Work out the finished part from the listing and answer in its coordinate system (mm). A direction names the side the tool comes from. Coordinates: 2 decimals unless noted, no trailing zeros. Loops run counter-clockwise (first coordinate to the right, second up) from the corner with the lowest first, then second, coordinate; pieces in that order, holes last. Notation, with made-up numbers: (47, 16) -> (84, 16) arc R21 cw to (84, 43) -> close; hole circle Ø10 at (-40, -4). An arc over 180 degrees is marked (long way). Answer as CSV lines item,"result".
Autodesk Inventor part; units mm, degrees
ref_plane "YZ Plane" through (0, 0, 0) normal (1, 0, 0) x (0, 1, 0)
ref_plane "XZ Plane" through (0, 0, 0) normal (0, 1, 0) x (-1, 0, 0)
ref_plane "XY Plane" through (0, 0, 0) normal (0, 0, 1) x (1, 0, 0)
sketch "Sketch1" plane through (0, 0, 0) normal (0, 1, 0) x (-1, 0, 0)
  circle A0 centre (26.4627, 138.7343) radius 5
  circle A1 centre (79.388, 116.8119) radius 5
  arc A2 (96.3331, 96.3331) -> (82.5566, 108.3722) centre (0, 0) ccw
  line L0 (82.5566, 108.3722) -> (85.4769, 112.4329)
  arc A3 (85.4769, 112.4329) -> (73.0752, 120.8614) centre (79.388, 116.8119) ccw
  line L1 (73.0752, 120.8614) -> (70.3746, 116.6514)
  arc A4 (70.3746, 116.6514) -> (32.7226, 132.2473) centre (0, 0) ccw
  line L2 (32.7226, 132.2473) -> (33.7899, 137.1339)
  arc A5 (33.7899, 137.1339) -> (19.0608, 139.9434) centre (26.4627, 138.7343) ccw
  line L3 (19.0608, 139.9434) -> (18.2544, 135.007)
  arc A6 (18.2544, 135.007) -> (0, 136.2355) centre (0, 0) ccw
  line L4 (0, 136.2355) -> (0, 134.2355)
  arc A7 (94.9189, 94.9189) -> (0, 134.2355) centre (0, 0) ccw
  line L5 (94.9189, 94.9189) -> (96.3331, 96.3331)
extrude "Extrusion1" add sketch "Sketch1" along normal blind 30 contours A0 | A1 | L5 A7 L4 A6 L3 A5 L2 A4 L1 A3 L0 A2
sketch "Sketch2" plane through (0, 30, 0) normal (0, 1, 0) x (1, 0, 0)
  arc A0 (-96.3331, -96.3331) -> (-82.5566, -108.3722) centre (0, 0) ccw
  line L0 (-82.5566, -108.3722) -> (-85.4769, -112.4329)
  arc A1 (-85.4769, -112.4329) -> (-73.0752, -120.8614) centre (-79.388, -116.8119) ccw
  line L1 (-73.0752, -120.8614) -> (-70.3746, -116.6514)
  arc A2 (-70.3746, -116.6514) -> (-32.7226, -132.2473) centre (0, 0) ccw
  line L2 (-32.7226, -132.2473) -> (-33.7899, -137.1339)
  arc A3 (-33.7899, -137.1339) -> (-19.0608, -139.9434) centre (-26.4627, -138.7343) ccw
  line L3 (-19.0608, -139.9434) -> (-18.2544, -135.007)
  arc A4 (-18.2544, -135.007) -> (0, -136.2355) centre (0, 0) ccw
  line L4 (0, -136.2355) -> (0, -134.2355)
  arc A5 (-94.9189, -94.9189) -> (0, -134.2355) centre (0, 0) ccw
  line L5 (-94.9189, -94.9189) -> (-96.3331, -96.3331)
  circle A6 centre (0, 0) radius 136.2355
  point P0 (0, 0)
  point P1 (-82.5566, -108.3722)
extrude "Extrusion2" cut sketch "Sketch2" against normal blind 20 contours A6 L1 A1 L0 | A6 L3 A3 L2
sketch "Sketch3" plane through (0, 0, 0) normal (0, -1, 0) x (1, 0, 0)
  arc A0 (-82.5566, 108.3722) -> (-96.3331, 96.3331) centre (0, 0) ccw
  line L0 (-94.9189, 94.9189) -> (-96.3331, 96.3331)
  arc A1 (0, 134.2355) -> (-94.9189, 94.9189) centre (0, 0) ccw
  line L1 (0, 136.2355) -> (0, 134.2355)
  arc A2 (0, 136.2355) -> (-18.2544, 135.007) centre (0, 0) ccw
  line L2 (-19.0608, 139.9434) -> (-18.2544, 135.007)
  arc A3 (-19.0608, 139.9434) -> (-33.7899, 137.1339) centre (-26.4627, 138.7343) ccw
  line L3 (-32.7226, 132.2473) -> (-33.7899, 137.1339)
  arc A4 (-32.7226, 132.2473) -> (-70.3746, 116.6514) centre (0, 0) ccw
  line L4 (-73.0752, 120.8614) -> (-70.3746, 116.6514)
  arc A5 (-73.0752, 120.8614) -> (-85.4769, 112.4329) centre (-79.388, 116.8119) ccw
  line L5 (-82.5566, 108.3722) -> (-85.4769, 112.4329)
  circle A6 centre (-26.4627, 138.7343) radius 4.75
  circle A7 centre (-79.388, 116.8119) radius 4.75
  point P0 (0, 0)
  dimension "d7" = 9.5
  dimension "d8" = 9.5
extrude "Extrusion3" cut sketch "Sketch3" against normal blind 10 contours A6 | A7
fillet "Fillet1" radius 1 4 edges at (0, 15, 136.2355) (0, 15, 134.2355) (-96.3331, 15, 96.3331) (-94.9189, 15, 94.9189)
sketch "Sketch4" plane through (0, 0, 0) normal (0, -1, 0) x (1, 0, 0)
  circle A0 centre (-26.4627, 138.7343) radius 4.75
  circle A1 centre (-26.4627, 138.7343) radius 5.25
  circle A2 centre (-79.388, 116.8119) radius 4.75
  circle A3 centre (-79.388, 116.8119) radius 5.25
  point P0 (0, 0)
  dimension "d12" = 10.5
  dimension "d15" = 10.5
extrude "Extrusion4" cut sketch "Sketch4" against normal blind 1 contours A1 | A2 | A3
properties part number "wall_standard"
(1) A cutting plane is placed at C-C, the plane z = 131. Write down the section's boundary in (x, y), and give its area (3 significant figures).
Computed values:
outline,"(-37.4, 0) -> (-29.29, 0) -> (-29.29, 30) -> (-37.4, 30) -> close"
area,"243 mm2"
(2) Flat-ended cylindrical pins translate along their axes: pin 1 Ø6 at (y, z) = (25, 117) entering from -X; pin 2 Ø12 at (y, z) = (23, 129) entering from +X; pin 3 Ø8 at (x, y) = (-76, 13.5) entering from -Z; pin 4 Ø6.5 at (x, z) = (-26.46, 138.73) entering from +Y. Find the tip coordinate at first contact, or state that the pin passes through.
Computed values:
pin 1,"x = -74.59"
pin 2,"x = -0.03"
pin 3,"z = 107.79"
pin 4,"through"
(3) Consider line 1 along X through (y, z) = (8.5, 140); line 2 along Y through (x, z) = (-32.5, 136); line 3 along Z through (x, y) = (-71, 24.25). Determine where each line is inside the solid, lowest interval first.
Computed values:
line 1,"-33.86 to -31.04, -21.88 to -19.07"
line 2,"0 to 10"
line 3,"113.92 to 116.27"
(4) Which of the six approach directions +Z, -Z, +X, -X, +Y, -Y give full straight-line access (tool end or side, diameter ignored) to faces 5 (the face through (-18.663, 4.93, 137.51)), 6 (the face through (-33.25, 4.93, 134.66)), 7 (the face through (-81, 10, 122))?
Computed values:
face 5,"+Z, +Y, -Y"
face 6,"-X, +Y, -Y"
face 7,"+Z, -X, +Y"
(5) For a pull along X with two mould halves and no side action, classify faces 1 (the face through (-27.7, 4.93, 146.13)), 2 (the face through (-28, 1, 134)), 3 (the face through (-51.87, 14.79, 125.975)), 4 (the face through (-51, 0, 125)) as pulls with the +X half, pulls with the -X half, needs draft (parallel to the pull), parting line crosses it, or undercut.
Computed values:
face 1,"parting line crosses it"
face 2,"undercut"
face 3,"undercut"
face 4,"needs draft"
(6) A cutting plane is placed at B-B, the plane x = -28. Write down the section's boundary in (y, z) (3 decimals).
Computed values:
outline,"(0, 131.283) -> (30, 131.283) -> (30, 133.327) -> (10, 133.327) -> (10, 134.24) -> (1, 134.24) -> (1, 133.714) -> (0, 133.714) -> close; (0, 143.754) -> (1, 143.754) -> (1, 143.229) -> (10, 143.229) -> (10, 146.075) -> (0, 146.075) -> close"
(7) A cutting plane is placed at A-A, the plane y = 7.75. Count the separate pieces of the cut face and the enclosed holes in it, and give its area (3 significant figures).
Computed values:
separate pieces,"1"
enclosed holes,"2"
area,"397 mm2"
